```python
from build123d import *

# Parameters (mm, degrees)
PAD028_DEPTH = 1.4
SKETCH048_R  = 1.75
PAD029_DEPTH = 1
PAD030_DEPTH = 1
PAD031_DEPTH = 1


with BuildPart() as part:
    # Sketch047 (on Face725 of Binder021) → Pad028 (new body)
    with BuildSketch(Plane(origin=(0, 135.8, 0), x_dir=(-1, 0, 0), z_dir=(0, 1, 0))):
        with BuildLine():
            Line((-120.499982, -0.1), (-120.499982, -26.3))
            Line((-120.499982, -26.3), (-68.48194, -26.3))
            ThreePointArc((-67.46705, -26.3), (-67.974495, -21.15), (-68.48194, -26.3))
            Line((-67.46705, -26.3), (-32.299995, -26.3))
            Line((-32.299995, -15.934266), (-32.299995, -26.3))
            ThreePointArc((-31.615729, -15.25), (-32.099578, -15.450417), (-32.299995, -15.934266))
            Line((-31.615729, -15.25), (-23.784261, -15.25))
            ThreePointArc((-23.099995, -15.934266), (-23.300412, -15.450417), (-23.784261, -15.25))
            Line((-23.099995, -15.934266), (-23.099995, -26.3))
            Line((-7.299995, -26.3), (-23.099995, -26.3))
            Line((-7.299995, -26.3), (-7.299995, -0.1))
            Line((-7.299995, -0.1), (-120.499982, -0.1))
        make_face()
        with BuildLine():
            Line((-105.199995, -19.86), (-92.199994, -19.86))
            ThreePointArc((-90.899995, -21.16), (-91.280756, -20.240762), (-92.199994, -19.86))
            Line((-90.899995, -21.16), (-90.899995, -24.776619))
            Line((-90.899995, -24.776619), (-91.938732, -25.120886))
            Line((-91.938732, -25.120886), (-92.869018, -25.773985))
            ThreePointArc((-93.61597, -26.01), (-93.224294, -25.949593), (-92.869018, -25.773985))
            Line((-93.61597, -26.01), (-103.78402, -26.01))
            ThreePointArc((-104.530977, -25.773981), (-104.175699, -25.949592), (-103.78402, -26.01))
            Line((-105.461258, -25.120886), (-104.530977, -25.773981))
            Line((-106.499995, -24.776619), (-105.461258, -25.120886))
            Line((-106.499995, -21.16), (-106.499995, -24.776619))
            ThreePointArc((-105.199995, -19.86), (-106.119234, -20.240761), (-106.499995, -21.16))
        make_face(mode=Mode.SUBTRACT)
    extrude(amount=-PAD028_DEPTH)

    # Sketch048 (on Face5 of Binder022) → Pad029 (join)
    with BuildSketch(Plane.XY.offset(-26.3)):
        with BuildLine():
            Line((18.199995, 134.4), (8.199995, 134.4))
            Line((8.199995, 134.4), (8.199995, 124.1))
            Line((8.199995, 124.1), (13.199995, 124.1))
            ThreePointArc((13.199995, 124.1), (16.735529, 125.564466), (18.199995, 129.1))
            Line((18.199995, 134.4), (18.199995, 129.1))
        make_face()
        with Locations((13.199995, 129.1)):
            Circle(SKETCH048_R, mode=Mode.SUBTRACT)
        with BuildLine():
            Line((109.449995, 134.4), (119.599982, 134.4))
            Line((119.599982, 134.4), (119.599982, 124.35))
            Line((119.599982, 124.35), (114.449995, 124.35))
            ThreePointArc((109.449995, 129.35), (110.914461, 125.814466), (114.449995, 124.35))
            Line((109.449995, 134.4), (109.449995, 129.35))
        make_face()
        with Locations((114.449995, 129.35)):
            Circle(SKETCH048_R, mode=Mode.SUBTRACT)
    extrude(amount=PAD029_DEPTH)

    # Sketch049 (on Face25 of Pad029) → Pad030 (join)
    with BuildSketch(Plane(origin=(8.199995, 0, 0), x_dir=(0, -1, 0), z_dir=(-1, 0, 0))):
        Polygon((-134.4, -25.3), (-124.1, -25.3), (-134.4, -15), align=None)
    extrude(amount=-PAD030_DEPTH)

    # Sketch050 (on Face36 of Pad030) → Pad031 (join)
    with BuildSketch(Plane.YZ.offset(119.599982)):
        Polygon((124.35, -25.3), (134.4, -25.3), (134.4, -15.25), align=None)
    extrude(amount=-PAD031_DEPTH)


solid = part.part
```
The model under review builds one solid part; all positions refer to its coordinate system, in mm. A direction names the side the tool comes from. Round coordinates to 2 decimals unless told otherwise and drop trailing zeros. Order: outer loops, then holes, each group sorted by start corner. A loop starts at its lowest first (then second) coordinate and runs counter-clockwise, first axis right, second up. Notation, with made-up numbers: (-16, 87) -> (40, 87) arc R36 cw to (40, 123) -> close; hole circle Ø3 at (-7, 71). An arc over 180 degrees is marked (long way). One line per item, written item: value. Start each with the question number.
Q1. Take a section at A-A (y = 133). Write out the cut boundary in (x, z), and give its area (3 significant figures).
Q2. Mouldability with a two-part tool opening along X and no side actions: class faces 4 (the face through (119.6, 130, -22)), 5 (the face through (119.11, 129.45, -20.2)), 6 (the face through (113, 131, -25.3)) as released by +X, released by -X, zero draft, split by the parting line, or undercut.
Q3. Wall thickness on line 1 (X direction, y = 134.95, z = -23.75); line 2 (Y direction, x = 22, z = -10); line 3 (Z direction, x = 30.5, y = 135.25): over which ranges is each line inside the solid? List them lowest first.
Q4. Take a section at D-D (z = -23.75). Write out the cut boundary in (x, y), and give its area (3 significant figures).
Q5. Take a section at B-B (z = -17.5). Write out the cut boundary in (x, y).
Q6. Clearance check with flat-ended pins moving along their axes: pin 1 Ø2.5 at (x, y) = (115, 131.5) entering from +Z; pin 2 Ø3 at (y, z) = (131, -18.5) entering from -X; pin 3 Ø3 at (y, z) = (128, -23.5) entering from +X; pin 4 Ø8.5 at (x, z) = (67.97, -23.75) entering from +Y. State where each tip first meets the part, or that it passes through.
Q7. Machinability: for faces 1 (the face through (8.2, 130, -22)), 2 (the face through (16.7, 125.53, -25.81)), 3 (the face through (15, 130, -25.3)), which of the approach directions +Z, -Z, +X, -X, +Y, -Y give a long, thin tool a straight path to every point of the face, cutting with its end or side? Answer none if there is none.
Q8. Take a section at C-C (x = 95). Write out the cut boundary in (y, z), and give its area (3 significant figures).
Reported:
1. outline: (8.2, -26.3) -> (18.2, -26.3) -> (18.2, -25.3) -> (9.2, -25.3) -> (9.2, -16.4) -> (8.2, -16.4) -> close; (109.45, -26.3) -> (119.6, -26.3) -> (119.6, -16.65) -> (118.6, -16.65) -> (118.6, -25.3) -> (109.45, -25.3) -> close
1. area: 37.7 mm2
2. face 4: released by +X
2. face 5: zero draft
2. face 6: undercut
3. line 1: x = 7.3 to 23.1, 32.3 to 65.37, 70.57 to 90.9, 106.5 to 120.5
3. line 2: y = 134.4 to 135.8
3. line 3: z = -15.25 to -0.1
4. outline: (7.3, 134.4) -> (8.2, 134.4) -> (8.2, 125.65) -> (9.2, 125.65) -> (9.2, 134.4) -> (23.1, 134.4) -> (23.1, 135.8) -> (7.3, 135.8) -> close; (32.3, 134.4) -> (65.37, 134.4) -> (65.37, 135.8) -> (32.3, 135.8) -> close; (70.57, 134.4) -> (90.9, 134.4) -> (90.9, 135.8) -> (70.57, 135.8) -> close; (106.5, 134.4) -> (118.6, 134.4) -> (118.6, 125.9) -> (119.6, 125.9) -> (119.6, 134.4) -> (120.5, 134.4) -> (120.5, 135.8) -> (106.5, 135.8) -> close
4. area: 134 mm2
5. outline: (7.3, 134.4) -> (8.2, 134.4) -> (8.2, 131.9) -> (9.2, 131.9) -> (9.2, 134.4) -> (23.1, 134.4) -> (23.1, 135.8) -> (7.3, 135.8) -> close; (32.3, 134.4) -> (118.6, 134.4) -> (118.6, 132.15) -> (119.6, 132.15) -> (119.6, 134.4) -> (120.5, 134.4) -> (120.5, 135.8) -> (32.3, 135.8) -> close
6. pin 1: stops at z = -25.3
6. pin 2: stops at x = 8.2
6. pin 3: stops at x = 119.6
6. pin 4: stops at y = 135.8
7. face 1: +Z, -Z, -X, -Y
7. face 2: +Z, -Z, -Y
7. face 3: +Z, -Y
8. outline: (134.4, -26.3) -> (135.8, -26.3) -> (135.8, -26.01) -> (134.4, -26.01) -> close; (134.4, -19.86) -> (135.8, -19.86) -> (135.8, -0.1) -> (134.4, -0.1) -> close
8. area: 28.1 mm2
